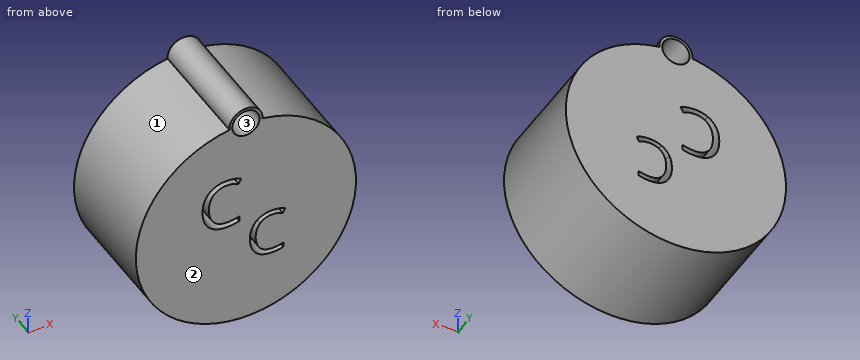
```python
from build123d import *

# Parameters (mm, degrees)
F0_R     = 3.1220096901
F1_DEPTH = 25.4


with BuildPart() as f1:
    # F0 (on Front) → F1 (new body)
    with BuildSketch(Plane.XZ):
        with BuildLine():
            ThreePointArc((3.762887104, 24.7915036788), (0, 21.3018608193), (-3.762887104, 24.7915036788))
            ThreePointArc((-3.762887104, 24.7915036788), (0, -25.0754456394), (3.762887104, 24.7915036788))
        make_face()
        with BuildLine():
            add(Edge.make_bspline(
                [(8.4130730817, -1.6073568671), (7.2075554314, -1.0429237476), (6.0020377811, -1.0429237476)],
                knots=[0, 0, 0, 1, 1, 1], degree=2))
            add(Edge.make_bspline(
                [(6.0020377811, -1.0429237476), (4.2529919416, -1.0429237476), (3.2402642046, -2.2077929222)],
                knots=[0, 0, 0, 1, 1, 1], degree=2))
            add(Edge.make_bspline(
                [(3.2402642046, -2.2077929222), (2.2275364675, -3.3726620968), (2.2275364675, -5.3981175709)],
                knots=[0, 0, 0, 1, 1, 1], degree=2))
            add(Edge.make_bspline(
                [(2.2275364675, -5.3981175709), (2.2275364675, -7.479319526), (3.204261269, -8.6163154601)],
                knots=[0, 0, 0, 1, 1, 1], degree=2))
            add(Edge.make_bspline(
                [(3.204261269, -8.6163154601), (4.1809860704, -9.7533113943), (5.9881011609, -9.7533113943)],
                knots=[0, 0, 0, 1, 1, 1], degree=2))
            add(Edge.make_bspline(
                [(5.9881011609, -9.7533113943), (7.0983852396, -9.7533113943), (8.5222432735, -9.3537949476)],
                knots=[0, 0, 0, 1, 1, 1], degree=2))
            Line((8.5222432735, -9.3537949476), (8.5222432735, -10.4338830157))
            add(Edge.make_bspline(
                [(8.5222432735, -10.4338830157), (7.418927505, -10.8496588527), (5.7999567877, -10.8496588527)],
                knots=[0, 0, 0, 1, 1, 1], degree=2))
            add(Edge.make_bspline(
                [(5.7999567877, -10.8496588527), (3.4562818182, -10.8496588527), (2.1822424518, -9.4258008188)],
                knots=[0, 0, 0, 1, 1, 1], degree=2))
            add(Edge.make_bspline(
                [(2.1822424518, -9.4258008188), (0.9082030853, -8.0019427848), (0.9082030853, -5.3818581807)],
                knots=[0, 0, 0, 1, 1, 1], degree=2))
            add(Edge.make_bspline(
                [(0.9082030853, -5.3818581807), (0.9082030853, -3.741982533), (1.5214143756, -2.5085916423)],
                knots=[0, 0, 0, 1, 1, 1], degree=2))
            add(Edge.make_bspline(
                [(1.5214143756, -2.5085916423), (2.134625666, -1.2752007515), (3.2925265305, -0.6074043652)],
                knots=[0, 0, 0, 1, 1, 1], degree=2))
            add(Edge.make_bspline(
                [(3.2925265305, -0.6074043652), (4.450427395, 0.060392021), (6.0182971714, 0.060392021)],
                knots=[0, 0, 0, 1, 1, 1], degree=2))
            add(Edge.make_bspline(
                [(6.0182971714, 0.060392021), (7.6860460595, 0.060392021), (8.9356963405, -0.5481737292)],
                knots=[0, 0, 0, 1, 1, 1], degree=2))
            Line((8.9356963405, -0.5481737292), (8.4130730817, -1.6073568671))
        make_face(mode=Mode.SUBTRACT)
        with BuildLine():
            add(Edge.make_bspline(
                [(-1.6337582686, 9.9965584062), (-2.9586341146, 10.6168759988), (-4.2835099606, 10.6168759988)],
                knots=[0, 0, 0, 1, 1, 1], degree=2))
            add(Edge.make_bspline(
                [(-4.2835099606, 10.6168759988), (-6.2057286735, 10.6168759988), (-7.318726494, 9.3366732305)],
                knots=[0, 0, 0, 1, 1, 1], degree=2))
            add(Edge.make_bspline(
                [(-7.318726494, 9.3366732305), (-8.4317243145, 8.0564704622), (-8.4317243145, 5.8304748212)],
                knots=[0, 0, 0, 1, 1, 1], degree=2))
            add(Edge.make_bspline(
                [(-8.4317243145, 5.8304748212), (-8.4317243145, 3.5432132451), (-7.3582940771, 2.2936434443)],
                knots=[0, 0, 0, 1, 1, 1], degree=2))
            add(Edge.make_bspline(
                [(-7.3582940771, 2.2936434443), (-6.2848638396, 1.0440736435), (-4.2988264443, 1.0440736435)],
                knots=[0, 0, 0, 1, 1, 1], degree=2))
            add(Edge.make_bspline(
                [(-4.2988264443, 1.0440736435), (-3.0786132374, 1.0440736435), (-1.5137791458, 1.4831461782)],
                knots=[0, 0, 0, 1, 1, 1], degree=2))
            Line((-1.5137791458, 1.4831461782), (-1.5137791458, 0.2961186862))
            add(Edge.make_bspline(
                [(-1.5137791458, 0.2961186862), (-2.7263341108, -0.1608230796), (-4.5055989752, -0.1608230796)],
                knots=[0, 0, 0, 1, 1, 1], degree=2))
            add(Edge.make_bspline(
                [(-4.5055989752, -0.1608230796), (-7.0813209956, -0.1608230796), (-8.4815028868, 1.4040110121)],
                knots=[0, 0, 0, 1, 1, 1], degree=2))
            add(Edge.make_bspline(
                [(-8.4815028868, 1.4040110121), (-9.8816847779, 2.9688451038), (-9.8816847779, 5.8483440522)],
                knots=[0, 0, 0, 1, 1, 1], degree=2))
            add(Edge.make_bspline(
                [(-9.8816847779, 5.8483440522), (-9.8816847779, 7.6505836423), (-9.2077594921, 9.0060924558)],
                knots=[0, 0, 0, 1, 1, 1], degree=2))
            add(Edge.make_bspline(
                [(-9.2077594921, 9.0060924558), (-8.5338342063, 10.3616012693), (-7.2612896799, 11.0955161166)],
                knots=[0, 0, 0, 1, 1, 1], degree=2))
            add(Edge.make_bspline(
                [(-7.2612896799, 11.0955161166), (-5.9887451534, 11.8294309638), (-4.2656407295, 11.8294309638)],
                knots=[0, 0, 0, 1, 1, 1], degree=2))
            add(Edge.make_bspline(
                [(-4.2656407295, 11.8294309638), (-2.4327681719, 11.8294309638), (-1.0593901273, 11.1606111726)],
                knots=[0, 0, 0, 1, 1, 1], degree=2))
            Line((-1.0593901273, 11.1606111726), (-1.6337582686, 9.9965584062))
        make_face(mode=Mode.SUBTRACT)
        with BuildLine():
            ThreePointArc((3.7735848201, 25.0754456394), (-0.1420717056, 28.8463550821), (-3.762887104, 24.7915036788))
            ThreePointArc((-3.762887104, 24.7915036788), (0, 21.3018608193), (3.762887104, 24.7915036788))
            ThreePointArc((3.762887104, 24.7915036788), (3.7709094427, 24.9333739338), (3.7735848201, 25.0754456394))
        make_face()
        with Locations((0, 25.0754456394)):
            Circle(F0_R, mode=Mode.SUBTRACT)
    extrude(amount=F1_DEPTH)


solid = f1.part
```
Check sheet for the modelled part. Datum: model origin and axes. Units: mm. Face numbers are marked on the shaded views. Coordinates: 2 decimals unless noted, no trailing zeros. Loops run counter-clockwise (first coordinate to the right, second up) from the corner with the lowest first, then second, coordinate; pieces in that order, holes last.
1) Gauge pin test, flat ends, axial feed: pin 1 (6 mm diameter, centred on y = -3, z = 15.5, fed in from -X); pin 2 (1.5 mm diameter, centred on y = -20.5, z = 12, fed in from -X); pin 3 (5 mm diameter, centred on y = -2.5, z = 6, fed in from -X). Record the tip position at first contact, or that the pin passes through.
2) Sectioned sample at D-D (x = -17.5). Record the boundary of the cut face in (y, z), and give its area (3 significant figures).
3) Sectioned sample at B-B (x = 7.5). Count the separate pieces of the cut face and the enclosed holes in it, and give its area (3 significant figures).
4) Release check for a two-part mould opening along X. For the marked faces 1, 2 and 3 record: released by +X, released by -X, zero draft, split by the parting line, or undercut.
5) Material ranges on probe 1 along Z at (x, y) = (0, -14.5); probe 2 along Z at (x, y) = (7, -19.75); probe 3 along Z at (x, y) = (4, -4.75), recorded low to high.
6) Sectioned sample at A-A (x = 0). Record the boundary of the cut face in (y, z).
Check sheet entries:
1. pin 1: stops at x = -21.74
1. pin 2: stops at x = -22.41
1. pin 3: stops at x = -24.83
2. outline: (-25.4, -17.96) - (0, -17.96) - (0, 17.96) - (-25.4, 17.96) - close
2. area: 912 mm2
3. separate pieces: 3
3. enclosed holes: 0
3. area: 1,160 mm2
4. face 1: split by the parting line
4. face 2: zero draft
4. face 3: undercut
5. probe 1: z = -25.08 to 21.95, 28.2 to 28.85
5. probe 2: z = -24.08 to -10.78, -9.68 to -1.14, 0 to 24.08
5. probe 3: z = -24.75 to -10.59, -9.28 to -1.56, -0.28 to 24.75
6. outline: (-25.4, -25.08) - (0, -25.08) - (0, 21.95) - (-25.4, 21.95) - close; (-25.4, 28.2) - (0, 28.2) - (0, 28.85) - (-25.4, 28.85) - close
